Part model, mm, in its own coordinate system. Face numbers are marked on the shaded views. Give positions to 0.01 mm unless a question says otherwise; leave off trailing zeros. Write each loop counter-clockwise with the first axis right and the second up, starting at its lowest first coordinate (ties: lowest second). Pieces come first, ordered by that corner, then holes.
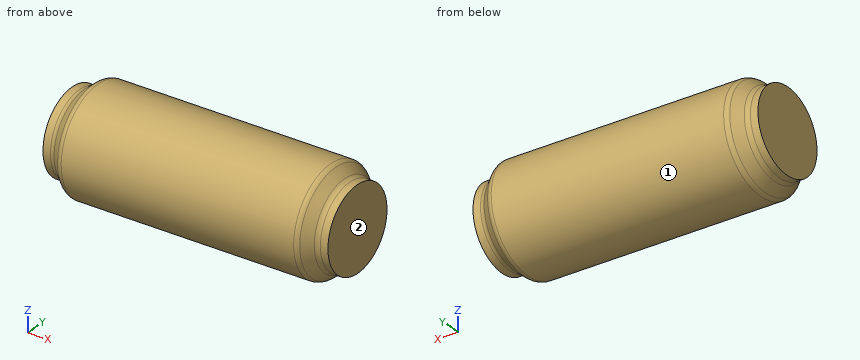
```python
from build123d import *


with BuildPart() as part:
    # Sketch1 → Revolve1 (revolve)
    with BuildSketch(Plane(origin=(0, 0, 0), x_dir=(1, 0, 0), z_dir=(0, 1, 0)), mode=Mode.PRIVATE) as revolve1_sk:
        with BuildLine():
            Line((95, 0), (95, 27.5))
            Line((95, 27.5), (90, 27.5))
            ThreePointArc((90, 27.5), (88.27509592, 27.80695132), (86.761976473, 28.690117634))
            Line((86.761976473, 28.690117634), (80.738023527, 33.809882366))
            ThreePointArc((80.738023527, 33.809882366), (79.22490408, 34.69304868), (77.5, 35))
            Line((77.5, 35), (-77.5, 35))
            ThreePointArc((-77.5, 35), (-79.22490408, 34.69304868), (-80.738023527, 33.809882366))
            Line((-80.738023527, 33.809882366), (-86.761976473, 28.690117634))
            ThreePointArc((-86.761976473, 28.690117634), (-88.27509592, 27.80695132), (-90, 27.5))
            Line((-90, 27.5), (-95, 27.5))
            Line((-95, 27.5), (-95, 0))
            Line((-95, 0), (95, 0))
        make_face()
    revolve(revolve1_sk.sketch.rotate(Axis((-95, 0, 0), (1, 0, 0)), 180), axis=Axis((-95, 0, 0), (1, 0, 0)))


solid = part.part
```
1) Saw through at C-C, the plane x = -67. Write the cut outline in (y, z).
Answers follow:
outline: circle Ø70 at (0, 0)
2) Saw through at A-A, the plane z = 0. Write the cut outline in (x, y), then the cut area to 3 significant figures.
Answers follow:
outline: (-95, -27.5) - (-90, -27.5) arc R5 cw to (-86.76, -28.69) - (-80.74, -33.81) arc R5 ccw to (-77.5, -35) - (77.5, -35) arc R5 ccw to (80.74, -33.81) - (86.76, -28.69) arc R5 cw to (90, -27.5) - (95, -27.5) - (95, 27.5) - (90, 27.5) arc R5 cw to (86.76, 28.69) - (80.74, 33.81) arc R5 ccw to (77.5, 35) - (-77.5, 35) arc R5 ccw to (-80.74, 33.81) - (-86.76, 28.69) arc R5 cw to (-90, 27.5) - (-95, 27.5) - close
area: 13,000 mm2
3) Pin check, flat tips, straight feed: pin 1 Ø8 at (x, z) = (-22.5, 5) entering from +Y; pin 2 Ø12 at (x, z) = (28.5, 10) entering from -Y; pin 3 Ø3 at (x, z) = (51, -1.5) entering from -Y. Stop position of each tip, or through.
Answers follow:
pin 1: stops at y = 34.99
pin 2: stops at y = -34.77
pin 3: stops at y = -35
4) Wall check: L1, parallel to Y at x = -22, z = 0.5; L2, parallel to Y at x = 8.5, z = 9; L3, parallel to Z at x = 3, y = -1. Give the ranges that are in metal, low to high.
Answers follow:
L1: y = -35 to 35
L2: y = -33.82 to 33.82
L3: z = -34.99 to 34.99
5) Two-plate mould, pull along Y, no slides. Class the marked faces 1 and 2: +Y half, -Y half, draft (parallel to the pull), parting line (faces both ways), or undercut.
Answers follow:
face 1: parting line
face 2: draft
